Autodesk Fusion 360 part; units mm, degrees
sketch "スケッチ1" plane through (0, 0, 0) normal (0, 0, 1) x (1, 0, 0)
  circle A0 centre (0, 0) radius 50
  dimension "d1" = 100
extrude "押し出し1" add sketch "スケッチ1" along normal blind 5
sketch "スケッチ2" plane through (0, 0, 5) normal (0, 0, 1) x (-1, 0, 0)
  circle A0 centre (0, 0) radius 50
  circle A1 centre (0, 0) radius 9
  circle A2 centre (0, 0) radius 6
  dimension "d4" = 18
  dimension "d5" = 12
extrude "押し出し2" add sketch "スケッチ2" along normal blind 25 contours A1
sketch "スケッチ3" plane through (0, 0, 0) normal (0, 1, 0) x (1, 0, 0)
  line L0 (9, -5) -> (9, -10)
  line L1 (9, -5) -> (19, -5)
  line L2 (19, -5) -> (9, -10)
revolve "回転1" add sketch "スケッチ3" angle 360 about axis through (0, 0, 1.75) along (0, 0, 1)
chamfer "面取り1" distance 0.5 angle 45 3 edges at (-46.6164, -18.0808, 0) (-46.6164, -18.0808, 5) (8.3909, 3.2545, 30)
sketch "スケッチ4" plane through (0, 0, 0) normal (0, 1, 0) x (1, 0, 0)
  line L0 (0, -30) -> (0, -25)
  line L1 (0, -10) -> (0, -15)
  circle A0 centre (0, -25) radius 1
  circle A1 centre (0, -15) radius 1
  dimension "d10" = 2
  dimension "d11" = 2
extrude "押し出し3" cut sketch "スケッチ4" along normal blind 9 and the other way blind 9
sketch "スケッチ5" plane through (0, 0, 0) normal (0, 0, 1) x (1, 0, 0)
  circle A0 centre (0, -40) radius 1.5
  circle A1 centre (-0.2424, -30) radius 1.5
  circle A2 centre (0, -20) radius 1.5
  point P0 (0, -20)
  point P1 (0, -30)
  point P2 (0, -40)
  dimension "d16" = 3
  dimension "d17" = 3
  dimension "d18" = 3
extrude "押し出し4" cut sketch "スケッチ5" along normal blind 6
pattern_circular "C パターン1" count 6 over 360 about axis through (0, 0, 1.75) along (0, 0, 1) of "押し出し4"
sketch "スケッチ6" plane through (0, 0, 0) normal (0, 0, 1) x (1, 0, 0)
  circle A0 centre (0, 0) radius 1.5
  dimension "d23" = 3
extrude "押し出し5" cut sketch "スケッチ6" along normal blind 5
sketch "スケッチ7" plane through (0, 0, 5) normal (0, 0, 1) x (-1, 0, 0)
  circle A0 centre (26.1019, 14.7901) radius 1.5
  circle A1 centre (25.8596, -15.2099) radius 1.5
  circle A2 centre (-0.2424, -30) radius 1.5
  circle A3 centre (-26.1019, -14.7901) radius 1.5
  circle A4 centre (-25.8596, 15.2099) radius 1.5
  circle A5 centre (34.641, 20) radius 1.5
  circle A6 centre (34.641, -20) radius 1.5
  circle A7 centre (0, -40) radius 1.5
  circle A8 centre (-34.641, -20) radius 1.5
  circle A9 centre (-34.641, 20) radius 1.5
  arc A10 (16.9721, 8.541) -> (15.8828, 10.4277) centre (17.3205, 10) ccw
  arc A11 (16.9721, -8.541) -> (16.9721, 8.541) centre (0, 0) ccw
  arc A12 (15.8828, -10.4277) -> (16.9721, -8.541) centre (17.3205, -10) ccw
  arc A13 (1.0893, -18.9688) -> (15.8828, -10.4277) centre (0, 0) ccw
  arc A14 (-1.0893, -18.9688) -> (1.0893, -18.9688) centre (0, -20) ccw
  arc A15 (-15.8828, -10.4277) -> (-1.0893, -18.9688) centre (0, 0) ccw
  arc A16 (-16.9721, -8.541) -> (-15.8828, -10.4277) centre (-17.3205, -10) ccw
  arc A17 (-16.9721, 8.541) -> (-16.9721, -8.541) centre (0, 0) ccw
  arc A18 (-15.8828, 10.4277) -> (-16.9721, 8.541) centre (-17.3205, 10) ccw
  arc A19 (-1.0893, 18.9688) -> (-15.8828, 10.4277) centre (0, 0) ccw
  arc A20 (1.0893, 18.9688) -> (-1.0893, 18.9688) centre (0, 20) ccw
  arc A21 (15.8828, 10.4277) -> (1.0893, 18.9688) centre (0, 0) ccw
  circle A22 centre (0.2424, 30) radius 1.5
  circle A23 centre (0, 40) radius 1.5
  circle A24 centre (0, 0) radius 49.5
  circle A25 centre (0, 20) radius 2.5
  circle A26 centre (-17.3205, 10) radius 2.5
  circle A27 centre (-17.3205, -10) radius 2.5
  circle A28 centre (0, -20) radius 2.5
  circle A29 centre (17.3205, -10) radius 2.5
  circle A30 centre (17.3205, 10) radius 2.5
  dimension "d26" = 5
  dimension "d28" = 360
extrude "押し出し6" cut sketch "スケッチ7" along normal blind 1 contours A10 A11 A21 A30 | A11 A12 A13 A29 | A19 A20 A21 A25 | A13 A14 A15 A28 | A17 A18 A19 A26 | A15 A16 A17 A27 picked at (15.697, 11.2338) picked at (15.697, -11.2338) picked at (0.2115, 19.7656) picked at (-1.8808, -19.2124) picked at (-15.6988, 11.2358) picked at (-17.2117, -9.7715)
Geometry: final body of the model. Coordinates: model frame, mm. Give positions to 0.01 mm unless a question says otherwise; leave off trailing zeros. Loops run counter-clockwise (first coordinate to the right, second up) from the corner with the lowest first, then second, coordinate; pieces in that order, holes last. Notation, with made-up numbers: (26, 19) - (36, 19) arc R23 ccw to (36, 33) - close; hole circle Ø3 at (20, -10). An arc over 180 degrees is marked (long way). One line per question, with ' | ' between items. Start each with the question number.
(1) Pull-direction query (Y, two-part tool) for faces 1 (the cylindrical face through (1.172, 8.923, 19.614)), 2 (the flat face through (-2, -6, 30)), 3 (the cylindrical face through (35.75, -18.99, 2.46)); classes: released by +Y, released by -Y, zero draft, split by the parting line, or undercut.
(2) Section query A-A on y = 0. Return loops of the section in (x, z).
(3) Contact query for flat-ended pins moving along their axis: pin 1 (5 mm diameter, centred on x = -17.32, y = 10, fed in from +Z); pin 2 (8 mm diameter, centred on y = -4, z = 16, fed in from +X); pin 3 (12 mm diameter, centred on x = 15.5, y = -19, fed in from +Z). Output: stop coordinate, or through.
(4) Section query B-B on z = 17.5. Return loops of the section in (x, y), then the cut area to 3 significant figures.
(5) Ray query, line 1 (X direction, y = -16, z = 3); line 2 (Y direction, x = 0, z = 10); line 3 (Z direction, x = -38, y = -31). Return the intervals inside material, ascending. Write a range as from..to.
The answers:
1) face 1: split by the parting line | face 2: zero draft | face 3: undercut
2) outline: (-50, 0.5) - (-49.5, 0) - (-1.5, 0) - (-1.5, 5) - (-6, 5) - (-6, 30) - (-8.5, 30) - (-9, 29.5) - (-9, 10) - (-19, 5) - (-49.5, 5) - (-50, 4.5) - close; (1.5, 0) - (49.5, 0) - (50, 0.5) - (50, 4.5) - (49.5, 5) - (19, 5) - (9, 10) - (9, 29.5) - (8.5, 30) - (6, 30) - (6, 5) - (1.5, 5) - close
3) pin 1: z = 5.75 | pin 2: x = 9 | pin 3: z = 5.24
4) outline: circle Ø18 at (0, 0); hole circle Ø12 at (0, 0) | area: 141 mm2
5) line 1: -47.37..-26.99, -25.22..24.58, 27.13..47.37 | line 2: -9..-6, 6..9 | line 3: 0..5
